from build123d import *

# Parameters (mm, degrees)
F0_R     = 19.05
F0_R_2   = 12.7
F1_DEPTH = 50.8
F2_R     = 27.305
F3_DEPTH = 12.7
F4_DEPTH = 42.750418


with BuildPart() as f1:
    # F0 (on Front) → F1 (new body)
    with BuildSketch(Plane.XZ):
        Circle(F0_R)
        Circle(F0_R_2, mode=Mode.SUBTRACT)
    extrude(amount=F1_DEPTH)

    # F2 (on Front) → F3 (join)
    with BuildSketch(Plane.XZ):
        Circle(F2_R)
    extrude(amount=F3_DEPTH)

    # F0 (on Front) → F4 (cut)
    with BuildSketch(Plane.XZ):
        Circle(F0_R_2)
    extrude(amount=F4_DEPTH, mode=Mode.SUBTRACT)


solid = f1.part
Read the model definition and answer for the solid it produces. Units are mm, in the model's axes. A direction names the side the tool comes from. Round coordinates to 2 decimals unless told otherwise and drop trailing zeros. Order: outer loops, then holes, each group sorted by start corner. A loop starts at its lowest first (then second) coordinate and runs counter-clockwise, first axis right, second up.
1) The part is cut by section A-A on z = 0. Write down the section's boundary in (x, y) (3 decimals).
2) The part is cut by section D-D on y = -8. Write down the section's boundary in (x, z) (3 decimals), plus the area to 3 significant figures.
3) Flat-ended cylindrical pins translate along their axes: pin 1 (10 mm diameter, centred on x = 11.5, y = -33, fed in from -Z); pin 2 (8 mm diameter, centred on y = -13.5, z = -20, fed in from +X); pin 3 (4 mm diameter, centred on x = 17, z = -20, fed in from -Y). Find the tip coordinate at first contact, or state that the pin passes through.
4) The part is cut by section B-B on x = 0. Write down the section's boundary in (y, z) (3 decimals).
5) Straight lines are drawn through the part: L1, parallel to Z at x = 0, y = -38.5; L2, parallel to Y at x = -22, z = 12.5; L3, parallel to Z at x = -3, y = -18. For each, find the intervals that lie inside material, in ascending order.
6) The part is cut by section C-C on y = -15. Write down the section's boundary in (x, z), plus the area to 3 significant figures.
7) For faces 1 (the face through (-15.12, -31.48, -11.59)), 2 (the face through (4, -50.8, -12.4)), determine the directions among +Z, -Z, +X, -X, +Y, -Y from which every point of the face is accessible in a straight line to the end or side of a thin tool.
Resolved:
1. outline: (-27.305, -12.7) - (-19.05, -12.7) - (-19.05, -50.8) - (-12.7, -50.8) - (-12.7, 0) - (-27.305, 0) - close; (12.7, -50.8) - (19.05, -50.8) - (19.05, -12.7) - (27.305, -12.7) - (27.305, 0) - (12.7, 0) - close
2. outline: circle Ø54.61 at (0, 0); hole circle Ø25.4 at (0, 0)
2. area: 1,840 mm2
3. pin 1: stops at z = -17.91
3. pin 2: stops at x = 22.07
3. pin 3: stops at y = -12.7
4. outline: (-50.8, -19.05) - (-12.7, -19.05) - (-12.7, -27.305) - (0, -27.305) - (0, -12.7) - (-50.8, -12.7) - close; (-50.8, 12.7) - (0, 12.7) - (0, 27.305) - (-12.7, 27.305) - (-12.7, 19.05) - (-50.8, 19.05) - close
5. L1: z = -19.05 to -12.7, 12.7 to 19.05
5. L2: y = -12.7 to 0
5. L3: z = -18.81 to -12.34, 12.34 to 18.81
6. outline: circle Ø38.1 at (0, 0); hole circle Ø25.4 at (0, 0)
6. area: 633 mm2
7. face 1: -Y
7. face 2: +Z, -Z, +X, -X, -Y
